from build123d import *

# Parameters (mm, degrees)
F0_W     = 2.54
F0_H     = 8.7372876405
F0_H_2   = 8.89
F1_DEPTH = 6.9977
F2_R     = 11.176
F3_DEPTH = 6.9977


with BuildPart() as f1:
    # F0 (on Top) → F1 (new body)
    with BuildSketch(Plane.XY):
        Polygon((-11.6335226281, 5.2501477372), (-10.3635226281, 7.4498522628), (-14.0807527651, 9.595996083), (-15.3507527651, 7.3962915574), align=None)
        Polygon((-15.3507527651, 7.3962915574), (-14.0807527651, 9.595996083), (-12.3768237899, 12.5472876405), (-14.124837026, 15.5749353777), (-14.2130055479, 15.7276477372), (-15.394837026, 17.7746399033), (-17.1428502621, 20.8022876405), (-26.6749032064, 20.8022876405), (-31.4409296786, 12.5472876405), (-26.6749032064, 4.2922876405), (-23.2670452561, 4.2922876405), (-20.7270452561, 4.2922876405), (-17.1428502621, 4.2922876405), align=None)
        Polygon((-18.7559669142, 18.0082876405), (-15.6030570942, 12.5472876405), (-18.7559669142, 7.0862876405), (-25.0617865543, 7.0862876405), (-28.2146963743, 12.5472876405), (-25.0617865543, 18.0082876405), align=None, mode=Mode.SUBTRACT)
        Polygon((14.2130055479, 9.6723522628), (10.3635226281, 7.4498522628), (11.6335226281, 5.2501477372), (15.4830055479, 7.4726477372), align=None)
        Polygon((-10.3635226281, -7.4498522628), (-11.6335226281, -5.2501477372), (-15.4830055479, -7.4726477372), (-14.2130055479, -9.6723522628), align=None)
        Polygon((-14.2130055479, 15.7276477372), (-14.124837026, 15.5749353777), (-6.4258711864, 20.0199353777), (-7.6958711864, 22.2196399033), (-15.394837026, 17.7746399033), align=None)
        Polygon((12.4649923118, 12.7), (14.2130055479, 9.6723522628), (15.4830055479, 7.4726477372), (17.231018784, 4.445), (20.7270452561, 4.445), (23.2670452561, 4.445), (26.7630717283, 4.445), (31.5290982004, 12.7), (26.7630717283, 20.955), (17.231018784, 20.955), (15.4830055479, 17.9273522628), (14.2130055479, 15.7276477372), align=None)
        Polygon((25.1499550762, 7.239), (18.8441354361, 7.239), (15.691225616, 12.7), (18.8441354361, 18.161), (25.1499550762, 18.161), (28.3028648962, 12.7), align=None, mode=Mode.SUBTRACT)
        Polygon((-14.2130055479, -9.6723522628), (-15.4830055479, -7.4726477372), (-17.231018784, -4.445), (-20.7270452561, -4.445), (-23.2670452561, -4.445), (-26.7630717283, -4.445), (-31.5290982004, -12.7), (-26.7630717283, -20.955), (-17.231018784, -20.955), (-15.4830055479, -17.9273522628), (-14.2130055479, -15.7276477372), (-12.4649923118, -12.7), align=None)
        Polygon((-25.1499550762, -7.239), (-18.8441354361, -7.239), (-15.691225616, -12.7), (-18.8441354361, -18.161), (-25.1499550762, -18.161), (-28.3028648962, -12.7), align=None, mode=Mode.SUBTRACT)
        with Locations((-21.9970452561, -0.0763561798)):
            Rectangle(F0_W, F0_H)
        Polygon((-7.6958711864, 22.2196399033), (-6.4258711864, 20.0199353777), (-4.6778579503, 16.9922876405), (-1.27, 16.9922876405), (1.27, 16.9922876405), (4.854194994, 16.9922876405), (6.6462924911, 20.0962915574), (7.9162924911, 22.295996083), (9.6202214662, 25.2472876405), (4.854194994, 33.5022876405), (-4.6778579503, 33.5022876405), (-9.4438844224, 25.2472876405), align=None)
        Polygon((6.3939514928, 25.2687924658), (3.2596837324, 19.7970718096), (-3.0460992385, 19.7755669843), (-6.217614449, 25.2257828151), (-3.0833466886, 30.6975034713), (3.2224362823, 30.7190082967), align=None, mode=Mode.SUBTRACT)
        Polygon((15.4830055479, -7.4726477372), (11.6335226281, -5.2501477372), (10.3635226281, -7.4498522628), (14.2130055479, -9.6723522628), align=None)
        Polygon((6.6462924911, 20.0962915574), (14.2130055479, 15.7276477372), (15.4830055479, 17.9273522628), (7.9162924911, 22.295996083), align=None)
        Polygon((17.231018784, -4.445), (15.4830055479, -7.4726477372), (14.2130055479, -9.6723522628), (12.4649923118, -12.7), (14.2130055479, -15.7276477372), (15.4830055479, -17.9273522628), (17.231018784, -20.955), (26.7630717283, -20.955), (31.5290982004, -12.7), (26.7630717283, -4.445), (23.2670452561, -4.445), (20.7270452561, -4.445), align=None)
        Polygon((18.8441354361, -18.161), (15.691225616, -12.7), (18.8441354361, -7.239), (25.1499550762, -7.239), (28.3028648962, -12.7), (25.1499550762, -18.161), align=None, mode=Mode.SUBTRACT)
        with Locations((21.9970452561, 0)):
            Rectangle(F0_W, F0_H_2)
        Polygon((-6.5140397082, -20.1726477372), (-14.2130055479, -15.7276477372), (-15.4830055479, -17.9273522628), (-7.7840397082, -22.3723522628), align=None)
        Polygon((-4.7660264722, -17.145), (-6.5140397082, -20.1726477372), (-7.7840397082, -22.3723522628), (-9.5320529443, -25.4), (-4.7660264722, -33.655), (4.7660264722, -33.655), (9.5320529443, -25.4), (7.7840397082, -22.3723522628), (6.5140397082, -20.1726477372), (4.7660264722, -17.145), (1.27, -17.145), (-1.27, -17.145), align=None)
        Polygon((-6.3058196401, -25.4), (-3.15290982, -19.939), (3.15290982, -19.939), (6.3058196401, -25.4), (3.15290982, -30.861), (-3.15290982, -30.861), align=None, mode=Mode.SUBTRACT)
        Polygon((15.4830055479, -17.9273522628), (14.2130055479, -15.7276477372), (6.5140397082, -20.1726477372), (7.7840397082, -22.3723522628), align=None)
    extrude(amount=F1_DEPTH)

    # F2 (on Top) → F3 (join)
    with BuildSketch(Plane.XY):
        Polygon((7.6989658396, 13.335), (-7.6989658396, 13.335), (-15.3979316793, 0), (-7.6989658396, -13.335), (7.6989658396, -13.335), (15.3979316793, 0), align=None)
        Circle(F2_R, mode=Mode.SUBTRACT)
    extrude(amount=F3_DEPTH)


solid = f1.part
Read the model definition and answer for the solid it produces. Units are mm, in the model's axes. A direction names the side the tool comes from. Coordinates: 2 decimals unless noted, no trailing zeros. Write each loop counter-clockwise with the first axis right and the second up, starting at its lowest first coordinate (ties: lowest second). Pieces come first, ordered by that corner, then holes. Notation, with made-up numbers: (-5.5, 15.5) -> (9.5, 15.5) arc R30 cw to (9.5, 38.5) -> close; hole circle Ø3 at (88, 70.5). An arc over 180 degrees is marked (long way). Return JSON: item names as keys, results as strings.
(1) The part is cut by section A-A on x = 0. Give the vertices of the cut face in (y, z) (3 decimals).
Answers below:
{"outline": "(-33.655, 0) -> (-30.861, 0) -> (-30.861, 6.998) -> (-33.655, 6.998) -> close; (-19.939, 0) -> (-17.145, 0) -> (-17.145, 6.998) -> (-19.939, 6.998) -> close; (-13.335, 0) -> (-11.176, 0) -> (-11.176, 6.998) -> (-13.335, 6.998) -> close; (11.176, 0) -> (13.335, 0) -> (13.335, 6.998) -> (11.176, 6.998) -> close; (16.992, 0) -> (19.786, 0) -> (19.786, 6.998) -> (16.992, 6.998) -> close; (30.708, 0) -> (33.502, 0) -> (33.502, 6.998) -> (30.708, 6.998) -> close"}
(2) The part is cut by section D-D on z = 6. State how many separate pieces and enclosed holes the cut face has, then the cut area to 3 significant figures.
Answers below:
{"separate pieces": "1", "enclosed holes": "11", "area": "1,190 mm^2"}
(3) Consider line 1 along Y through (x, z) = (0, 4) (3 decimals); line 2 along Y through (x, z) = (22, 5) (3 decimals); line 3 along Y through (x, z) = (19, 6) (3 decimals). Determine where each line is inside the solid, lowest interval first. Write a range as from..to.
Answers below:
{"line 1": "-33.655..-30.861, -19.939..-17.145, -13.335..-11.176, 11.176..13.335, 16.992..19.786, 30.708..33.502", "line 2": "-20.955..-18.161, -7.239..7.239, 18.161..20.955", "line 3": "-20.955..-18.161, -7.239..-4.445, 4.445..7.239, 18.161..20.955"}
(4) The part is cut by section C-C on x = -18. Give the vertices of the cut face in (y, z) (3 decimals), then the cut area to 3 significant figures.
Answers below:
{"outline": "(-20.955, 0) -> (-16.699, 0) -> (-16.699, 6.998) -> (-20.955, 6.998) -> close; (-8.701, 0) -> (-4.445, 0) -> (-4.445, 6.998) -> (-8.701, 6.998) -> close; (4.292, 0) -> (8.396, 0) -> (8.396, 6.998) -> (4.292, 6.998) -> close; (16.699, 0) -> (20.802, 0) -> (20.802, 6.998) -> (16.699, 6.998) -> close", "area": "117 mm^2"}
(5) The part is cut by section B-B on y = -2.5. Give the vertices of the cut face in (x, z), then the cut area to 3 significant figures.
Answers below:
{"outline": "(-23.27, 0) -> (-20.73, 0) -> (-20.73, 7) -> (-23.27, 7) -> close; (-13.95, 0) -> (-10.89, 0) -> (-10.89, 7) -> (-13.95, 7) -> close; (10.89, 0) -> (13.95, 0) -> (13.95, 7) -> (10.89, 7) -> close; (20.73, 0) -> (23.27, 0) -> (23.27, 7) -> (20.73, 7) -> close", "area": "78.4 mm^2"}
(6) Each of these flat-tipped pins is pushed along its axis until it touches: P1, Ø3, axis at x = -23.5, z = 5, coming from the -Y side (3 decimals); P2, Ø3, axis at x = -8, z = 4, coming from the -Y side; P3, Ø3, axis at x = 24.5, z = 3, coming from the +Y side (3 decimals). Where does it stop, or does it pass through?
Answers below:
{"P1": "y = -20.955", "P2": "y = -30.65", "P3": "y = 20.955"}
(7) For a pull along X with two mould halves and no side action, classify faces 1 (the flat face through (29.11, -16.89, 3.45)), 2 (the flat face through (0, -33.655, 3)), 3 (the flat face through (12.54, -8.707, 3.45)) as pulls with the +X half, pulls with the -X half, needs draft (parallel to the pull), parting line crosses it, or undercut.
Answers below:
{"face 1": "pulls with the +X half", "face 2": "needs draft", "face 3": "undercut"}
(8) Which of the six approach directions +Z, -Z, +X, -X, +Y, -Y give full straight-line access (tool end or side, diameter ignored) to faces 4 (the flat face through (13.327, 11.207, 3.45)), 5 (the flat face through (8.756, 23.751, 3.45))?
Answers below:
{"face 4": "+Z, -Z", "face 5": "+Z, -Z, +X"}
